from build123d import *

# Parameters (mm, degrees)
SKETCH1_W                       = 25
SKETCH1_H                       = 6.75
BOSS_EXTRUDE1_DEPTH             = 6.5
BOSS_EXTRUDE4_DEPTH             = 6.5
BOSS_EXTRUDE3_REACH             = 6.85
BOSS_EXTRUDE3_DIRECTION_2_REACH = 6.85
SKETCH4_W                       = 2.3
SKETCH4_H                       = 4.5
CUT_EXTRUDE1_DEPTH              = 23
SKETCH6_R                       = 2.55
CUT_EXTRUDE2_DEPTH              = 10
BOSS_EXTRUDE5_DEPTH             = 1.475
CUT_EXTRUDE3_DEPTH              = 3
SKETCH9_R                       = 0.56
CUT_EXTRUDE4_DEPTH              = 9.7


with BuildPart() as part:
    # Sketch1 → Boss-Extrude1 (new body)
    with BuildSketch(Plane(origin=(0, 0, 0), x_dir=(1, 0, 0), z_dir=(0, 1, 0))):
        with Locations((12.5, -3.375)):
            Rectangle(SKETCH1_W, SKETCH1_H)
    extrude(amount=BOSS_EXTRUDE1_DEPTH)

    # Sketch5 → Boss-Extrude4 (add)
    with BuildSketch(Plane(origin=(0, 6.5, 0), x_dir=(1, 0, 0), z_dir=(0, 1, 0))):
        Polygon((-5.600297611, -3.375), (-2.800148806, -8.225), (2.800148806, -8.225), (5.600297611, -3.375), (2.800148806, 1.475), (-2.800148806, 1.475), align=None)
    extrude(amount=-BOSS_EXTRUDE4_DEPTH)

    # Boss-Extrude3: up to this face of the body (flat: up to its plane)
    boss_extrude3_end = Plane(part.part.faces().sort_by_distance((0, 3.25, -1.475))[0])
    # Sketch3 → Boss-Extrude3 (add, up to the picked face)
    with BuildSketch(Plane.XY.offset(3.375), mode=Mode.PRIVATE) as boss_extrude3_sk1:
        Polygon((21.275684175, 14.155521181), (26.183820092, 15.109566157), (30, -4.522977512), (25.091864083, -5.477022488), align=None)
    boss_extrude3_tool1 = split(extrude(boss_extrude3_sk1.sketch, amount=-BOSS_EXTRUDE3_REACH, mode=Mode.PRIVATE), bisect_by=boss_extrude3_end, keep=Keep.BOTH, mode=Mode.PRIVATE)
    add(boss_extrude3_tool1.solids().sort_by_distance((25.637842, 4.816272, 3.375))[0])

    # Boss-Extrude3 direction 2: up to this face of the body (flat: up to its plane)
    boss_extrude3_direction_2_end = Plane(part.part.faces().sort_by_distance((0, 3.25, 8.225))[0])
    # Sketch3 → Boss-Extrude3 direction 2 (add, up to the picked face)
    with BuildSketch(Plane.XY.offset(3.375), mode=Mode.PRIVATE) as boss_extrude3_direction_2_sk1:
        Polygon((21.275684175, 14.155521181), (26.183820092, 15.109566157), (30, -4.522977512), (25.091864083, -5.477022488), align=None)
    boss_extrude3_direction_2_tool1 = split(extrude(boss_extrude3_direction_2_sk1.sketch, amount=BOSS_EXTRUDE3_DIRECTION_2_REACH, mode=Mode.PRIVATE), bisect_by=boss_extrude3_direction_2_end, keep=Keep.BOTH, mode=Mode.PRIVATE)
    add(boss_extrude3_direction_2_tool1.solids().sort_by_distance((25.637842, 4.816272, 3.375))[0])

    # Sketch4 → Cut-Extrude1 (cut)
    with BuildSketch(Plane(origin=(-1.876769127, 9.65514015, 0), x_dir=(0.981627183, 0.190808995, 0), z_dir=(-0.190808995, 0.981627183, 0))):
        with Locations((27.435790708, -3.375)):
            Rectangle(SKETCH4_W, SKETCH4_H)
    extrude(amount=-CUT_EXTRUDE1_DEPTH, mode=Mode.SUBTRACT)

    # Sketch6 → Cut-Extrude2 (cut)
    with BuildSketch(Plane(origin=(0, 6.5, 0), x_dir=(1, 0, 0), z_dir=(0, 1, 0))):
        with Locations((0, -3.335615973)):
            Circle(SKETCH6_R)
    extrude(amount=-CUT_EXTRUDE2_DEPTH, mode=Mode.SUBTRACT)

    # Sketch7 → Boss-Extrude5 (add)
    with BuildSketch(Plane(origin=(0, 0, -1.475), x_dir=(-1, 0, 0), z_dir=(0, 0, -1))):
        Polygon((-2.800148806, 0), (-24.027238758, 0), (-25.091864083, -5.477022488), (-30, -4.522977512), (-26.183820092, 15.109566157), (-21.275684175, 14.155521181), (-22.763766749, 6.5), (-2.800148806, 6.5), align=None)
    extrude(amount=-BOSS_EXTRUDE5_DEPTH)

    # Sketch8 → Cut-Extrude3 (cut)
    with BuildSketch(Plane(origin=(0, 0, 0), x_dir=(-1, 0, 0), z_dir=(0, -1, 0))):
        Polygon((-4.67653718, -11.475), (4.67653718, -11.475), (9.353074361, -3.375), (4.67653718, 4.725), (-4.67653718, 4.725), (-9.353074361, -3.375), align=None)
    extrude(amount=-CUT_EXTRUDE3_DEPTH, mode=Mode.SUBTRACT)

    # Sketch9 → Cut-Extrude4 (cut)
    with BuildSketch(Plane(origin=(0, 0, -1.475), x_dir=(-1, 0, 0), z_dir=(0, 0, -1))):
        with Locations((-28.584915246, -3.269967081)):
            Circle(SKETCH9_R)
        with Locations((-27.917083762, 0.165728061)):
            Circle(SKETCH9_R)
    extrude(amount=-CUT_EXTRUDE4_DEPTH, mode=Mode.SUBTRACT)


solid = part.part
Verification items for the finished model (mm, model axes). A direction names the side the tool comes from. Give positions to 0.01 mm unless a question says otherwise; leave off trailing zeros. Write each loop counter-clockwise with the first axis right and the second up, starting at its lowest first coordinate (ties: lowest second). Pieces come first, ordered by that corner, then holes.
(1) Cross-section at A-A (x = 0). Enter the section's corners in (y, z) (3 decimals), plus the area to 3 significant figures.
(2) Cross-section at B-B (z = 4.5). Enter the section's corners in (x, y), plus the area to 3 significant figures.
(3) Material ranges on line 1 (Z direction, x = 27.5, y = 5) (3 decimals); line 2 (Y direction, x = 0, z = 6); line 3 (Y direction, x = 19, z = 2), recorded low to high.
(4) Mould release check, pull along X, two halves, no side actions. Record for faces 1 (the face through (28.477, 0.19, 6.907)), 2 (the face through (27, 5, 5.625)), 3 (the face through (3.22, 4.77, 7.5)), 4 (the face through (23.15, 14.52, 3.31)): +X half, -X half, draft (parallel to the pull), parting line (faces both ways), or undercut.
(5) Cross-section at C-C (y = 5). Enter the section's corners in (x, z) (3 decimals).
(6) Access from +Z, -Z, +X, -X, +Y, -Y to the whole of each face (thin tool, end or side, straight path). Record for faces 5 (the face through (15, 0, 3)), 6 (the face through (-4.181, 4.774, 0.916)), 7 (the face through (7.933, 1.479, 0.916)).
(7) Cross-section at D-D (y = 8.5). Enter the section's corners in (x, z) (3 decimals).
(8) Gauge pin test, flat ends, axial feed: pin 1 (3 mm diameter, centred on x = 4.5, z = 4.5, fed in from -Y); pin 2 (4 mm diameter, centred on x = 19, z = 3, fed in from -Y); pin 3 (1 mm diameter, centred on x = 16.5, z = 2.5, fed in from +Y); pin 4 (1 mm diameter, centred on x = 27.92, y = 0.17, fed in from -Z). Record the tip position at first contact, or that the pin passes through.
Worked out:
1. outline: (3, -1.475) - (6.5, -1.475) - (6.5, 0.786) - (3, 0.786) - close; (3, 5.886) - (6.5, 5.886) - (6.5, 8.225) - (3, 8.225) - close
1. area: 16.1 mm2
2. outline: (-4.95, 3) - (-2.27, 3) - (-2.27, 6.5) - (-4.95, 6.5) - close; (2.27, 3) - (8.7, 3) - (8.7, 0) - (24.03, 0) - (25.09, -5.48) - (27.74, -4.96) - (23.93, 14.67) - (21.28, 14.16) - (22.76, 6.5) - (2.27, 6.5) - close
2. area: 181 mm2
3. line 1: z = -1.475 to 1.125, 5.625 to 8.225
3. line 2: y = 3 to 6.5
3. line 3: y = 0 to 6.5
4. face 1: undercut
4. face 2: draft
4. face 3: undercut
4. face 4: -X half
5. outline: (-5.6, 3.375) - (-2.8, -1.475) - (28.149, -1.475) - (28.149, 1.125) - (25.806, 1.125) - (25.806, 5.625) - (28.149, 5.625) - (28.149, 8.225) - (23.055, 8.225) - (23.055, 6.75) - (3.652, 6.75) - (2.8, 8.225) - (-2.8, 8.225) - close; hole circle Ø5.1 at (0, 3.336)
6. face 5: +Z, -Z, -X, -Y
6. face 6: -Z, -X, +Y, -Y
6. face 7: -X, -Y
7. outline: (22.375, -1.475) - (27.469, -1.475) - (27.469, 1.125) - (25.126, 1.125) - (25.126, 5.625) - (27.469, 5.625) - (27.469, 8.225) - (22.375, 8.225) - close
8. pin 1: stops at y = 3
8. pin 2: stops at y = 0
8. pin 3: stops at y = 6.5
8. pin 4: passes through
